from build123d import *

# Parameters (mm, degrees)
F0_W      = 25.4
F0_H      = 69.85
F1_DEPTH  = 38.1
F2_W      = 44.45
F2_H      = 25.4
F3_DEPTH  = 25.4
F5_DEPTH  = 25.4
F7_DEPTH  = 25.4
F4_W      = 25.4
F4_H      = 25.4
F8_DEPTH  = 25.4
F9_R      = 6.35
F10_DEPTH = 76.2
F11_DEPTH = 25.4
F13_DEPTH = 25.4


with BuildPart() as f1:
    # F0 (on Top) → F1 (new body)
    with BuildSketch(Plane.XY):
        with Locations((12.7, 34.925)):
            Rectangle(F0_W, F0_H)
    extrude(amount=F1_DEPTH)

    # F2 (on face) → F3 (cut)
    with BuildSketch(Plane(origin=(0, 0, 0), x_dir=(0, -1, 0), z_dir=(-1, 0, 0))):
        with Locations((-22.225, 25.4)):
            Rectangle(F2_W, F2_H)
    extrude(amount=-F3_DEPTH, mode=Mode.SUBTRACT)

    # F2 (on face) → F5 (cut)
    with BuildSketch(Plane(origin=(0, 0, 0), x_dir=(0, -1, 0), z_dir=(-1, 0, 0))):
        with Locations((-22.225, 25.4)):
            Rectangle(F2_W, F2_H)
    extrude(amount=-F5_DEPTH, mode=Mode.SUBTRACT)

    # F6 (on face) → F7 (cut)
    with BuildSketch(Plane.XY.offset(38.1)):
        with BuildLine():
            ThreePointArc((0, 57.15), (3.7197438789, 66.1302561211), (12.7, 69.85))
            Line((12.7, 69.85), (0, 69.85))
            Line((0, 69.85), (0, 57.15))
        make_face()
        with BuildLine():
            ThreePointArc((12.7, 69.85), (21.6802561211, 66.1302561211), (25.4, 57.15))
            Line((25.4, 57.15), (25.4, 69.85))
            Line((25.4, 69.85), (12.7, 69.85))
        make_face()
        with BuildLine():
            Line((0, 44.45), (12.7, 44.45))
            ThreePointArc((12.7, 44.45), (3.7197438789, 48.1697438789), (0, 57.15))
            Line((0, 57.15), (0, 44.45))
        make_face()
        with BuildLine():
            Line((25.4, 44.45), (25.4, 57.15))
            ThreePointArc((25.4, 57.15), (21.6802561211, 48.1697438789), (12.7, 44.45))
            Line((12.7, 44.45), (25.4, 44.45))
        make_face()
    extrude(amount=-F7_DEPTH, mode=Mode.SUBTRACT)

    # F4 (on face) → F8 (cut)
    with BuildSketch(Plane.XY.offset(38.1)):
        with Locations((12.7, 57.15)):
            Rectangle(F4_W, F4_H)
    extrude(amount=F8_DEPTH, mode=Mode.SUBTRACT)

    # F9 (on face) → F10 (cut)
    with BuildSketch(Plane.XY.offset(38.1)):
        with Locations((12.7, 57.15)):
            Circle(F9_R)
    extrude(amount=-F10_DEPTH, mode=Mode.SUBTRACT)

    # F11 (cut): faces of the model
    f11_faces = [f1.faces().sort_by_distance(p)[0] for p in [
        (2.8367728246, 67.0132271754, 12.7),
        (22.5632271754, 67.0132271754, 12.7),
    ]]
    extrude(f11_faces, amount=-F11_DEPTH, mode=Mode.SUBTRACT)

    # F12 (on face) → F13 (cut)
    with BuildSketch(Plane.XY.offset(12.7)):
        with BuildLine():
            Line((6.35, 31.75), (19.05, 31.75))
            ThreePointArc((19.05, 31.75), (12.7, 38.1), (6.35, 31.75))
        make_face()
        with BuildLine():
            Line((19.05, 12.7), (19.05, 31.75))
            ThreePointArc((19.05, 31.75), (12.7, 25.4), (6.35, 31.75))
            Line((6.35, 31.75), (6.35, 12.7))
            ThreePointArc((6.35, 12.7), (12.7, 19.05), (19.05, 12.7))
        make_face()
        with BuildLine():
            ThreePointArc((6.35, 31.75), (12.7, 25.4), (19.05, 31.75))
            Line((19.05, 31.75), (6.35, 31.75))
        make_face()
        with BuildLine():
            ThreePointArc((6.35, 12.7), (12.7, 6.35), (19.05, 12.7))
            ThreePointArc((19.05, 12.7), (12.7, 19.05), (6.35, 12.7))
        make_face()
    extrude(amount=-F13_DEPTH, mode=Mode.SUBTRACT)


solid = f1.part
Could you check a few things on this model? Use its own coordinates, in mm. A direction names the side the tool comes from. Give positions to 0.01 mm unless a question says otherwise; leave off trailing zeros. Order: outer loops, then holes, each group sorted by start corner. A loop starts at its lowest first (then second) coordinate and runs counter-clockwise, first axis right, second up.
1. Which directions (+Z, -Z, +X, -X, +Y, -Y) give clear straight access to the entire face, cutting with the end or side of a thin tool? Please do faces 1 (the flat face through (13, 0, 6)), 2 (the cylindrical face through (12.56, 6.35, 6.44)).
Answers below:
face 1: +Z, -Z, +X, -X, -Y
face 2: +Z, -Z
2. I need wall thicknesses on L1, parallel to Y at x = 12.7, z = 11.5; L2, parallel to X at y = 20.5, z = 4. Which ranges of each line are inside material? Lowest first, please.
Answers below:
L1: y = 0 to 6.35, 38.1 to 50.8, 63.5 to 69.85
L2: x = 0 to 6.35, 19.05 to 25.4
3. Suppose I cut it at A-A (y = 19.5). Write out the boundary of the cut face in (x, z).
Answers below:
outline: (0, 0) - (6.35, 0) - (6.35, 12.7) - (0, 12.7) - close; (19.05, 0) - (25.4, 0) - (25.4, 12.7) - (19.05, 12.7) - close
4. Suppose I cut it at D-D (z = 28.5). Write out the boundary of the cut face in (x, y).
Answers below:
outline: circle Ø25.4 at (12.7, 57.15); hole circle Ø12.7 at (12.7, 57.15)
5. Suppose I cut it at C-C (z = 10.5). Write out the boundary of the cut face in (x, y), plus the area to 3 significant figures.
Answers below:
outline: (0, 0) - (25.4, 0) - (25.4, 57.15) arc R12.7 ccw to (0, 57.15) - close; hole (6.35, 12.7) arc R6.35 ccw to (19.05, 12.7) - (19.05, 31.75) arc R6.35 ccw to (6.35, 31.75) - close; hole circle Ø12.7 at (12.7, 57.15)
area: 1,210 mm2
6. Suppose I cut it at B-B (x = 12.7). Write out the boundary of the cut face in (y, z), plus the area to 3 significant figures.
Answers below:
outline: (0, 0) - (6.35, 0) - (6.35, 12.7) - (0, 12.7) - close; (38.1, 0) - (50.8, 0) - (50.8, 38.1) - (44.45, 38.1) - (44.45, 12.7) - (38.1, 12.7) - close; (63.5, 0) - (69.85, 0) - (69.85, 38.1) - (63.5, 38.1) - close
area: 645 mm2
7. For pin 1 (10 mm diameter, centred on y = 19.5, z = 5, fed in from -X); pin 2 (4 mm diameter, centred on x = 13, z = 20.5, fed in from -Y); pin 3 (3 mm diameter, centred on x = 7, z = 20.5, fed in from -Y); pin 4 (3 mm diameter, centred on y = 47, z = 18, fed in from -X), each with a flat end and sliding along its axis, tell me the tip position at first contact or that it passes through.
Answers below:
pin 1: stops at x = 0
pin 2: stops at y = 44.45
pin 3: stops at y = 45.16
pin 4: stops at x = 3.4
8. Thinking about a two-plate mould opening in X: for faces 3 (the cylindrical face through (12.142, 69.838, 23.55)), 4 (the flat face through (6.35, 22, 6)), 5 (the flat face through (4, 23, 12.7)), 6 (the flat face through (0, 28, 6)), which applies, +X half, -X half, draft (parallel to the pull), parting line (faces both ways), or undercut?
Answers below:
face 3: parting line
face 4: undercut
face 5: draft
face 6: -X half
